```python
from build123d import *

# Parameters (mm, degrees)
SKETCH1_R           = 19.05
SKETCH1_W           = 88.9
SKETCH1_H           = 88.9
BOSS_EXTRUDE1_DEPTH = 12.7
SKETCH2_W           = 76.2
SKETCH2_H           = 76.2
CUT_EXTRUDE1_DEPTH  = 2.54
SKETCH3_W           = 5.08
SKETCH3_H           = 3.81
SKETCH3_W_2         = 3.81
SKETCH3_H_2         = 5.08
SKETCH3_W_3         = 12.7
CUT_EXTRUDE2_DEPTH  = 2.54
SKETCH4_R           = 3.5
CUT_EXTRUDE4_DEPTH  = 5
FILLET8_R           = 0.508
FILLET9_R           = 2.54
FILLET10_R          = 0.508
FILLET11_R          = 1.27


with BuildPart() as part:
    # Sketch1 → Boss-Extrude1 (new body)
    with BuildSketch(Plane(origin=(0, 0, 0), x_dir=(1, 0, 0), z_dir=(0, 1, 0))):
        with BuildLine():
            ThreePointArc((-35.674486373, -7.268553459), (-40.384167339, 5.271691754), (-52.184486373, 11.61135385))
            Line((-52.184486373, 11.61135385), (-52.184486373, -26.148460768))
            ThreePointArc((-52.184486373, -26.148460768), (-40.384167339, -19.808798672), (-35.674486373, -7.268553459))
        make_face()
        with BuildLine():
            Line((-52.184486373, -26.148460768), (-52.184486373, 11.61135385))
            ThreePointArc((-52.184486373, 11.61135385), (-73.774486373, -7.268553459), (-52.184486373, -26.148460768))
        make_face()
        with Locations((39.255513627, -7.268553459)):
            Circle(SKETCH1_R)
        with Locations((-54.724486373, -7.268553459)):
            Circle(SKETCH1_R)
        with Locations((-7.734486373, -7.268553459)):
            Rectangle(SKETCH1_W, SKETCH1_H)
        with BuildLine():
            ThreePointArc((58.305513627, -7.268553459), (51.79575884, 7.071765575), (36.715513627, 11.61135385))
            Line((36.715513627, 11.61135385), (36.715513627, -26.148460768))
            ThreePointArc((36.715513627, -26.148460768), (51.79575884, -21.608872493), (58.305513627, -7.268553459))
        make_face()
        with BuildLine():
            Line((36.715513627, -26.148460768), (36.715513627, 11.61135385))
            ThreePointArc((36.715513627, 11.61135385), (20.205513627, -7.268553459), (36.715513627, -26.148460768))
        make_face()
    extrude(amount=BOSS_EXTRUDE1_DEPTH)

    # Sketch2 → Cut-Extrude1 (cut)
    with BuildSketch(Plane(origin=(0, 12.7, 0), x_dir=(1, 0, 0), z_dir=(0, 1, 0))):
        with Locations((-7.734486373, -7.268553459)):
            Rectangle(SKETCH2_W, SKETCH2_H)
    extrude(amount=-CUT_EXTRUDE1_DEPTH, mode=Mode.SUBTRACT)

    # Sketch3 → Cut-Extrude2 (cut)
    with BuildSketch(Plane(origin=(0, 12.7, 0), x_dir=(1, 0, 0), z_dir=(0, 1, 0))):
        with Locations((-61.074486373, -2.823553459)):
            Rectangle(SKETCH3_W, SKETCH3_H)
        with Locations((-65.519486373, -7.268553459)):
            Rectangle(SKETCH3_W_2, SKETCH3_H_2)
        with Locations((-61.074486373, -7.268553459)):
            Rectangle(SKETCH3_W, SKETCH3_H_2)
        with Locations((-56.629486373, -7.268553459)):
            Rectangle(SKETCH3_W_2, SKETCH3_H_2)
        with Locations((-61.074486373, -11.713553459)):
            Rectangle(SKETCH3_W, SKETCH3_H)
        with Locations((45.605513627, -7.268553459)):
            Rectangle(SKETCH3_W_3, SKETCH3_H_2)
    extrude(amount=-CUT_EXTRUDE2_DEPTH, mode=Mode.SUBTRACT)

    # Sketch4 → Cut-Extrude4 (cut)
    with BuildSketch(Plane.XZ):
        with Locations((-29.959486373, 7.268553459)):
            Circle(SKETCH4_R)
        with Locations((14.490513627, 7.268553459)):
            Circle(SKETCH4_R)
    extrude(amount=-CUT_EXTRUDE4_DEPTH, mode=Mode.SUBTRACT)

    # Fillet8
    fillet8_edges = [part.edges().sort_by_distance(p)[0] for p in [
        (-33.459486373, 0, 7.268553459),
        (10.990513627, 0, 7.268553459),
    ]]
    fillet(fillet8_edges, radius=FILLET8_R)

    # Fillet9
    fillet9_edges = [part.edges().sort_by_distance(p)[0] for p in [
        (-7.734486373, 12.7, 51.718553459),
        (-52.184486373, 6.35, -37.181446541),
        (36.715513627, 6.35, -37.181446541),
        (36.715513627, 6.35, 51.718553459),
        (-52.184486373, 6.35, 51.718553459),
        (36.715513627, 12.7, 38.933507114),
        (58.305513627, 12.7, 7.268553459),
        (36.715513627, 12.7, -24.396400195),
        (-7.734486373, 12.7, -37.181446541),
        (-52.184486373, 12.7, -24.396400195),
        (-73.774486373, 12.7, 7.268553459),
        (-52.184486373, 12.7, 38.933507114),
    ]]
    fillet(fillet9_edges, radius=FILLET9_R)

    # Fillet10
    fillet10_edges = [part.edges().sort_by_distance(p)[0] for p in [
        (-63.614486373, 12.7, 2.823553459),
        (-61.074486373, 12.7, 0.918553459),
        (-54.724486373, 12.7, 7.268553459),
        (-56.629486373, 12.7, 9.808553459),
        (-63.614486373, 12.7, 11.713553459),
        (-65.519486373, 12.7, 9.808553459),
        (-65.519486373, 12.7, 4.728553459),
        (-67.424486373, 12.7, 7.268553459),
        (-61.074486373, 12.7, 13.618553459),
        (-58.534486373, 12.7, 11.713553459),
        (-56.629486373, 12.7, 4.728553459),
        (-58.534486373, 12.7, 2.823553459),
        (51.955513627, 12.7, 7.268553459),
        (45.605513627, 12.7, 4.728553459),
        (39.255513627, 12.7, 7.268553459),
        (45.605513627, 12.7, 9.808553459),
    ]]
    fillet(fillet10_edges, radius=FILLET10_R)

    # Fillet11
    fillet11_edges = [part.edges().sort_by_distance(p)[0] for p in [
        (-45.834486373, 12.7, 7.268553459),
        (-7.734486373, 12.7, 45.368553459),
        (30.365513627, 12.7, 7.268553459),
        (-7.734486373, 12.7, -30.831446541),
    ]]
    fillet(fillet11_edges, radius=FILLET11_R)


solid = part.part
```
Here's how the part is built. I have some questions about the finished solid (model axes, mm). A direction names the side the tool comes from. Give positions to 0.01 mm unless a question says otherwise; leave off trailing zeros. Loops run counter-clockwise (first coordinate to the right, second up) from the corner with the lowest first, then second, coordinate; pieces in that order, holes last. Notation, with made-up numbers: M 52.25,6.5 L 95.25,6.5 A29 ccw 95.25,40.5 Z; hole C 76,84.5 d3. An arc over 180 degrees is marked long. Use one line per item in the form item = value. Start each with the question number.
Q1. I need wall thicknesses on line 1 along Z through (x, y) = (25, 10.5); line 2 along X through (y, z) = (1, -21.5); line 3 along Y through (x, z) = (10, 4.5). Which ranges of each line are inside material? Lowest first, please.
Q2. Thinking about a two-plate mould opening in X: for faces 4 (the flat face through (-8, 5, 51.719)), 5 (the cylindrical face through (35.952, 5.151, 50.994)), 6 (the flat face through (-8, 10.16, 7)), 7 (the cylindrical face through (-26.62, 2.72, 8.32)), which applies, +X half, -X half, draft (parallel to the pull), parting line (faces both ways), or undercut?
Q3. If we section it at B-B (x = 4): Write out the boundary of the cut face in (y, z), then the cut area to 3 significant figures.
Q4. If we section it at A-A (y = 7.25): Write out the boundary of the cut face in (x, z).
Q5. Will these pins go through, and if not, where does the flat tip stop? pin 1 Ø0.6 at (x, y) = (-66.5, 11) entering from -Z; pin 2 Ø1 at (y, z) = (11.5, -3) entering from +X; pin 3 Ø1 at (y, z) = (11.5, 8) entering from -X.
Q6. Which directions (+Z, -Z, +X, -X, +Y, -Y) give clear straight access to the entire face, cutting with the end or side of a thin tool? Please do faces 1 (the flat face through (14, 5, 7)), 2 (the flat face through (46, 10.16, 7)), 3 (the flat face through (-9, 0, 7)).
Taken from the geometry:
q1.line_1 = -37.16 to -30.83, 45.37 to 51.7
q1.line_2 = -52.18 to 36.72
q1.line_3 = 0 to 10.16
q2.face_4 = draft
q2.face_5 = +X half
q2.face_6 = undercut
q2.face_7 = undercut
q3.outline = M 0,-37.18 L 10.16,-37.18 A2.54 ccw 12.7,-34.64 L 12.7,-32.1 A1.27 ccw 11.43,-30.83 L 10.16,-30.83 L 10.16,45.37 L 11.43,45.37 A1.27 ccw 12.7,46.64 L 12.7,49.18 A2.54 ccw 10.16,51.72 L 0,51.72 Z
q3.area = 932 mm^2
q4.outline = M -52.18,-34.64 A2.54 ccw -49.64,-37.18 L 34.18,-37.18 A2.54 ccw 36.72,-34.64 L 36.72,-11.61 A19.05 ccw long 36.72,26.15 L 36.72,49.18 A2.54 ccw 34.18,51.72 L -49.64,51.72 A2.54 ccw -52.18,49.18 L -52.18,26.15 A19.05 ccw long -52.18,-11.61 Z
q5.pin_1 = -7.79
q5.pin_2 = 55.29
q5.pin_3 = -73.62
q6.face_1 = -Y
q6.face_2 = +Y
q6.face_3 = +Z, -Z, +X, -X, -Y
